```python
from build123d import *

# Parameters (mm, degrees)
SKETCH1_W           = 8
SKETCH1_H           = 8
SKETCH1_R           = 3
BOSS_EXTRUDE3_DEPTH = 15
CUT_EXTRUDE1_DEPTH  = 8
SKETCH4_W           = 8
SKETCH4_H           = 8.522050623
BOSS_EXTRUDE4_DEPTH = 10
SKETCH5_R           = 3
CUT_EXTRUDE2_DEPTH  = 10


with BuildPart() as part:
    # Sketch1 → Boss-Extrude3 (new body)
    with BuildSketch(Plane(origin=(0, 0, 0), x_dir=(1, 0, 0), z_dir=(0, 1, 0))):
        with Locations((4, 4)):
            Rectangle(SKETCH1_W, SKETCH1_H)
        with Locations(Location((3.995564868, 3.791433264, 0), (0, 0, 270))):
            Circle(SKETCH1_R, mode=Mode.SUBTRACT)
    extrude(amount=BOSS_EXTRUDE3_DEPTH)

    # Sketch3 → Cut-Extrude1 (cut)
    with BuildSketch(Plane.ZY):
        Polygon((-8, 15), (0, 15), (-8, 12.063105925), align=None)
    extrude(amount=-CUT_EXTRUDE1_DEPTH, mode=Mode.SUBTRACT)

    # Sketch4 → Boss-Extrude4 (add)
    with BuildSketch(Plane(origin=(0, 13.218525518, -4.852676159), x_dir=(1, 0, 0), z_dir=(0, 0.9387411967802677, -0.3446229323007264))):
        with Locations((4, -0.908318673)):
            Rectangle(SKETCH4_W, SKETCH4_H)
    extrude(amount=BOSS_EXTRUDE4_DEPTH)

    # Sketch5 → Cut-Extrude2 (cut)
    with BuildSketch(Plane(origin=(0, 22.605937486, -8.298905482), x_dir=(1, 0, 0), z_dir=(0, 0.9387411967802677, -0.34462293230072644))):
        with Locations((3.74552854, -2.73801251)):
            Circle(SKETCH5_R)
    extrude(amount=-CUT_EXTRUDE2_DEPTH, mode=Mode.SUBTRACT)


solid = part.part
```
Model file for the job. Use its own axes, mm. A direction names the side the tool comes from. Coordinates: 2 decimals unless noted, no trailing zeros. Order: outer loops, then holes, each group sorted by start corner. A loop starts at its lowest first (then second) coordinate and runs counter-clockwise, first axis right, second up. Notation, with made-up numbers: (-30.75, 41) - (17.25, 41) arc R15 cw to (17.25, 56) - close; hole circle Ø8 at (82.5, -12.5). An arc over 180 degrees is marked (long way). Return JSON: item names as keys, results as strings. Group by question number.
1) Tool access for faces 1 (the flat face through (6.73, 19.63, -1.7)), 2 (the cylindrical face through (4.9, 7.25, -0.93)): list every direction of +Z, -Z, +X, -X, +Y, -Y with a clear straight run to the whole face (end or side of a thin tool).
2) Saw through at A-A, the plane x = 1.25. Write the cut outline in (y, z).
3) Saw through at D-D, the plane z = -9.25. Write the cut outline in (x, y).
4) Probe line 1 (Z direction, x = 0.75, y = 10); line 2 (X direction, y = 21, z = -7.75); line 3 (Z direction, x = 2, y = 12.5). List the from-to ranges inside material, lowest first. Write a range as from..to.
5) Saw through at C-C, the plane x = 6.5. Write the cut outline in (y, z).
6) Saw through at B-B, the plane y = 7. Write the cut outline in (x, z).
7) Mould opens along X. For faces 3 (the flat face through (3.06, 14.74, -0.71)), 4 (the flat face through (8, 11, -4)), 5 (the flat face through (4, 6, -8)) say: released by +X, released by -X, zero draft, split by the parting line, or undercut.
8) Flat gauge pins, fed straight in: P1, Ø1, axis at x = 4, z = -1.5, coming from the +Y side; P2, Ø4, axis at x = 3, y = 7.5, coming from the -Z side; P3, Ø5, axis at y = 21.5, z = -2, coming from the -X side. Where does each tip first touch, or does it go through?
Values found:
{
 "1": {"face 1": "+Z, +X, -X, +Y", "face 2": "-Y"},
 "2": {"outline": "(0, -8) - (12.06, -8) - (21.45, -11.45) - (22.98, -7.29) - (13.59, -3.85) - (13.16, -5) - (0, -5) - close; (0, -2.58) - (14.05, -2.58) - (14.74, -0.72) - (24.12, -4.17) - (24.39, -3.45) - (15, 0) - (0, 0) - close"},
 "3": {"outline": "(0, 15.47) - (8, 15.47) - (8, 22.26) - (0, 22.26) - close"},
 "4": {"line 1": "z = -8..0", "line 2": "x = 0..2.61, 4.88..8", "line 3": "z = -8.16..-6.03, -1.55..0"},
 "5": {"outline": "(0, -8) - (12.06, -8) - (21.45, -11.45) - (23.14, -6.84) - (13.75, -3.4) - (13, -5.44) - (0, -5.44) - close; (0, -2.14) - (14.21, -2.14) - (14.57, -1.17) - (23.96, -4.61) - (24.39, -3.45) - (15, 0) - (0, 0) - close"},
 "6": {"outline": "(0, -8) - (8, -8) - (8, 0) - (0, 0) - close; hole circle Ø6 at (4, -3.79)"},
 "7": {"face 3": "undercut", "face 4": "released by +X", "face 5": "zero draft"},
 "8": {"P1": "passes through", "P2": "stops at z = -8", "P3": "stops at x = 0"}
}
